Could you check a few things on this model? Use its own coordinates, in mm. Coordinates: 2 decimals unless noted, no trailing zeros. Loops run counter-clockwise (first coordinate to the right, second up) from the corner with the lowest first, then second, coordinate; pieces in that order, holes last. Notation, with made-up numbers: (74, 60.25) -> (102, 60.25) arc R22 ccw to (102, 82.25) -> close; hole circle Ø11 at (27.5, 65.25). An arc over 180 degrees is marked (long way). One line per question, with ' | ' between items.
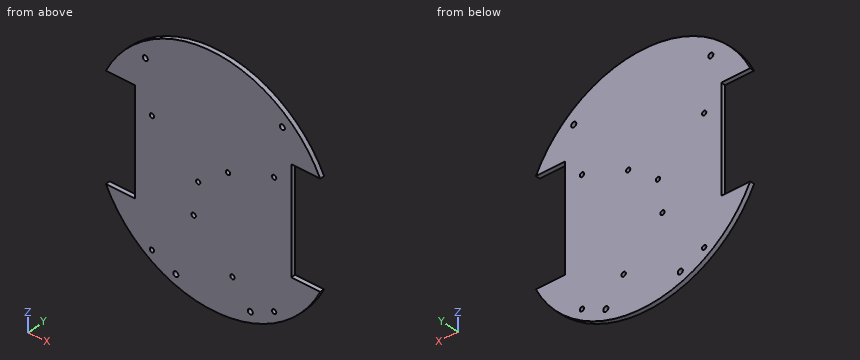
from build123d import *

# Parameters (mm, degrees)
ESQUISSE1_R             = 80
BOSS_EXTRU_1_DEPTH      = 3
ESQUISSE2_W             = 55
ESQUISSE2_H             = 70
ENL_V_MAT_EXTRU_1_DEPTH = 114.176852757
D_GAGEMENT_M2_51_D      = 2.9
D_GAGEMENT_M2_51_DEPTH  = 24
D_GAGEMENT_M2_51_TIP    = 0.871247898
D_GAGEMENT_M2_52_D      = 2.9
D_GAGEMENT_M2_52_DEPTH  = 24
D_GAGEMENT_M2_52_TIP    = 0.871247898
D_GAGEMENT_M31_D        = 3.4
D_GAGEMENT_M31_DEPTH    = 24
D_GAGEMENT_M31_TIP      = 1.021463052


with BuildPart() as part:
    # Esquisse1 → Boss.-Extru.1 (new body)
    with BuildSketch(Plane(origin=(0, 0, 0), x_dir=(1, 0, 0), z_dir=(0, 1, 0))):
        with Locations(Location((0, 0, 0), (0, 0, 270))):
            Circle(ESQUISSE1_R)
    extrude(amount=BOSS_EXTRU_1_DEPTH)

    # Esquisse2 → Enlèv. mat.-Extru.1 (cut, through all)
    with BuildSketch(Plane(origin=(0, 3, 0), x_dir=(1, 0, 0), z_dir=(0, 1, 0))):
        with Locations((-80, 0)):
            Rectangle(ESQUISSE2_W, ESQUISSE2_H)
        with Locations((80, 0)):
            Rectangle(ESQUISSE2_W, ESQUISSE2_H)
    extrude(amount=-ENL_V_MAT_EXTRU_1_DEPTH, mode=Mode.SUBTRACT)

    # Dégagement M2.51
    with Locations(Plane(origin=(0, 3, 0), x_dir=(1, 0, 0), z_dir=(0, 1, 0))):
        with Locations((-41, 61.5), (-41, -21.5), (41, -21.5), (41, 61.5)):
            Hole(D_GAGEMENT_M2_51_D / 2, depth=D_GAGEMENT_M2_51_DEPTH)
            with Locations((0, 0, -(D_GAGEMENT_M2_51_DEPTH + D_GAGEMENT_M2_51_TIP / 2))):  # 118° drill point
                Cone(0, D_GAGEMENT_M2_51_D / 2, D_GAGEMENT_M2_51_TIP, mode=Mode.SUBTRACT)

    # Dégagement M2.52
    with Locations(Plane(origin=(0, 3, 0), x_dir=(1, 0, 0), z_dir=(0, 1, 0))):
        with Locations((-13, 27), (13, 53), (-10, 5), (10, -10)):
            Hole(D_GAGEMENT_M2_52_D / 2, depth=D_GAGEMENT_M2_52_DEPTH)
            with Locations((0, 0, -(D_GAGEMENT_M2_52_DEPTH + D_GAGEMENT_M2_52_TIP / 2))):  # 118° drill point
                Cone(0, D_GAGEMENT_M2_52_D / 2, D_GAGEMENT_M2_52_TIP, mode=Mode.SUBTRACT)

    # Dégagement M31
    with Locations(Plane(origin=(0, 3, 0), x_dir=(1, 0, 0), z_dir=(0, 1, 0))):
        with Locations((-45.483572208, -55), (46.516427792, -55), (-25, 69), (25, 69)):
            Hole(D_GAGEMENT_M31_D / 2, depth=D_GAGEMENT_M31_DEPTH)
            with Locations((0, 0, -(D_GAGEMENT_M31_DEPTH + D_GAGEMENT_M31_TIP / 2))):  # 118° drill point
                Cone(0, D_GAGEMENT_M31_D / 2, D_GAGEMENT_M31_TIP, mode=Mode.SUBTRACT)


solid = part.part
1) I need wall thicknesses on line 1 along X through (y, z) = (2.1, -69); line 2 along X through (y, z) = (1.05, -5); line 3 along X through (y, z) = (1.5, 55). Which ranges of each line are inside material? Lowest first, please. Write a range as from..to.
Data:
line 1: -40.48..-26.7, -23.3..23.3, 26.7..40.48 | line 2: -52.5..-11.45, -8.55..52.5 | line 3: -58.09..-47.18, -43.78..44.82, 48.22..58.09
2) If we section it at D-D on z = -42: Please give me the cut outline in (x, y).
Data:
outline: (-68.09, 0) -> (68.09, 0) -> (68.09, 3) -> (-68.09, 3) -> close
3) If we section it at C-C on z = 14: Please give me the cut outline in (x, y).
Data:
outline: (-52.5, 0) -> (52.5, 0) -> (52.5, 3) -> (-52.5, 3) -> close
4) I'm going to push flat-ended pins straight in: pin 1 Ø4 at (x, z) = (-41, 21.5) entering from -Y; pin 2 Ø1.5 at (x, y) = (59, 2) entering from -Z; pin 3 Ø2.5 at (x, z) = (-13, -27) entering from -Y; pin 4 Ø1.5 at (x, y) = (-36.5, 0.5) entering from -Z. Where does each tip first touch, or does it pass through?
Data:
pin 1: y = 0 | pin 2: z = -54.84 | pin 3: through | pin 4: z = -71.57
5) If we section it at A-A on y = 1.7: Give the number of separate pieces and of enclosed holes in the cut face, and give its area (3 significant figures).
Data:
separate pieces: 1 | enclosed holes: 12 | area: 16,500 mm²
6) If we section it at B-B on x = 58.5: Please give me the cut outline in (y, z), and give its area (3 significant figures).
Data:
outline: (0, -54.57) -> (3, -54.57) -> (3, -35) -> (0, -35) -> close; (0, 35) -> (3, 35) -> (3, 54.57) -> (0, 54.57) -> close | area: 117 mm²
